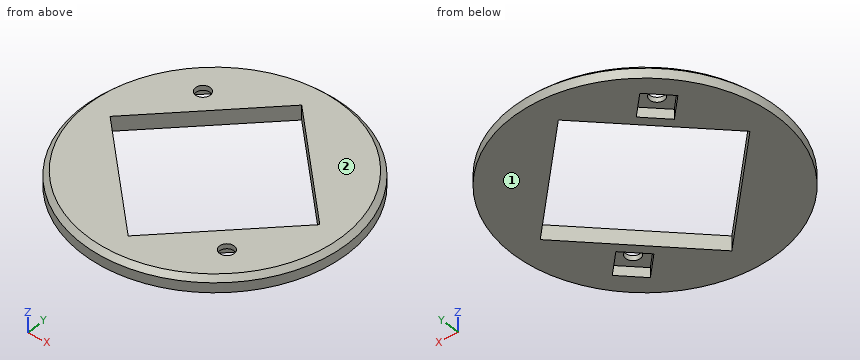
from build123d import *

# Parameters (mm, degrees)
BOX318_W                    = 6
BOX318_H                    = 6
BOX318_DEPTH                = 20
BOX318_PLACEMENT_ANGLE      = 45
BOX319_W                    = 6
BOX319_H                    = 6
BOX319_DEPTH                = 20
BOX319_PLACEMENT_ANGLE      = 135
CYLINDER809_R               = 1.5
CYLINDER809_DEPTH           = 20
CYLINDER809_PLACEMENT_ANGLE = 135
CYLINDER808_R               = 1.5
CYLINDER808_DEPTH           = 20
CYLINDER808_PLACEMENT_ANGLE = 45
BOX315_W                    = 30.2
BOX315_H                    = 30.2
BOX315_DEPTH                = 100
BOX315_PLACEMENT_ANGLE      = 45
CYLINDER805_R               = 27
CYLINDER805_DEPTH           = 3
CHAMFER_SIZE                = 1


with BuildPart() as krychle318:
    # Box318 → Box318 (new body)
    with BuildSketch(Plane.XY):
        with Locations((3, 3)):
            Rectangle(BOX318_W, BOX318_H)
    extrude(amount=BOX318_DEPTH)


with BuildPart() as krychle318_1:
    # Box318 placement: moved
    add(krychle318.part.moved(Location((9.899495, -14.142136, -30))).rotate(Axis((9.899495, -14.142136, -30), (0, 0, -1)), BOX318_PLACEMENT_ANGLE))


with BuildPart() as compound722:
    # Box319 → Box319 (new body)
    with BuildSketch(Plane.XY):
        with Locations((3, 3)):
            Rectangle(BOX319_W, BOX319_H)
    extrude(amount=BOX319_DEPTH)


with BuildPart() as compound722_1:
    # Box319 placement: moved
    add(compound722.part.moved(Location((-9.899495, 14.142136, -30))).rotate(Axis((-9.899495, 14.142136, -30), (0, 0, 1)), BOX319_PLACEMENT_ANGLE))

    # Compound722: union Krychle318
    add(krychle318_1.part)


with BuildPart() as compound722_2:
    # Compound722 placement: moved
    add(compound722_1.part.moved(Location((0, 0, -13))))


with BuildPart() as obj1:
    # Cylinder809 → Cylinder809 (new body)
    with BuildSketch(Plane.XY):
        Circle(CYLINDER809_R)
    extrude(amount=CYLINDER809_DEPTH)


with BuildPart() as obj1_1:
    # Cylinder809 placement: moved
    add(obj1.part.moved(Location((-14.142136, 14.142136, -30))).rotate(Axis((-14.142136, 14.142136, -30), (0, 0, 1)), CYLINDER809_PLACEMENT_ANGLE))


with BuildPart() as compound:
    # Cylinder808 → Cylinder808 (new body)
    with BuildSketch(Plane.XY):
        Circle(CYLINDER808_R)
    extrude(amount=CYLINDER808_DEPTH)


with BuildPart() as compound_1:
    # Cylinder808 placement: moved
    add(compound.part.moved(Location((14.142136, -14.142136, -30))).rotate(Axis((14.142136, -14.142136, -30), (0, 0, -1)), CYLINDER808_PLACEMENT_ANGLE))

    # Compound: union obj1
    add(obj1_1.part)


with BuildPart() as krychle315:
    # Box315 → Box315 (new body)
    with BuildSketch(Plane.XY):
        with Locations((15.1, 15.1)):
            Rectangle(BOX315_W, BOX315_H)
    extrude(amount=BOX315_DEPTH)


with BuildPart() as krychle315_1:
    # Box315 placement: moved
    add(krychle315.part.moved(Location((0, -21.354625, -30))).rotate(Axis((0, -21.354625, -30), (0, 0, 1)), BOX315_PLACEMENT_ANGLE))


with BuildPart() as cut344:
    # Cylinder805 → Cylinder805 (new body)
    with BuildSketch(Plane.XY.offset(-25)):
        Circle(CYLINDER805_R)
    extrude(amount=CYLINDER805_DEPTH)

    # Chamfer
    chamfer_edges = [cut344.edges().sort_by_distance(p)[0] for p in [
        (-27, 0, -22),
    ]]
    chamfer(chamfer_edges, length=CHAMFER_SIZE)

    # Cut340: cut Krychle315
    add(krychle315_1.part, mode=Mode.SUBTRACT)

    # Cut342: cut Compound
    add(compound_1.part, mode=Mode.SUBTRACT)

    # Cut344: cut Compound722
    add(compound722_2.part, mode=Mode.SUBTRACT)


solid = cut344.part
Geometry: final body of the model. Coordinates: model frame, mm. Face numbers are marked on the shaded views. Coordinates: 2 decimals unless noted, no trailing zeros. Order: outer loops, then holes, each group sorted by start corner. A loop starts at its lowest first (then second) coordinate and runs counter-clockwise, first axis right, second up. Notation, with made-up numbers: (-18.5, 27.25) - (29.5, 27.25) arc R16 cw to (29.5, 48.25) - close; hole circle Ø9 at (74, 86.5). An arc over 180 degrees is marked (long way). Use one line per item in the form item = value.
1) Ray query, L1, parallel to X at y = 13, z = -22.55; L2, parallel to X at y = 14, z = -24; L3, parallel to Y at x = 13, z = -23.6. Return the intervals inside material, ascending.
Solutions:
L1 = -23.15 to -15.11, -13.17 to -8.35, 8.35 to 23.15
L2 = -23.09 to -18.24, -10.04 to -7.35, 7.35 to 23.09
L3 = -23.66 to -17.24, -11.04 to -8.35, 8.35 to 23.66
2) Section A-A (z = -23.6). Return loops of the section in (x, y), then the cut area to 3 significant figures.
Solutions:
outline = circle Ø54 at (0, 0); hole (-21.35, 0) - (0, -21.35) - (21.35, 0) - (0, 21.35) - close; hole (-18.38, 14.14) - (-14.14, 9.9) - (-9.9, 14.14) - (-14.14, 18.38) - close; hole (9.9, -14.14) - (14.14, -18.38) - (18.38, -14.14) - (14.14, -9.9) - close
area = 1,310 mm^2
3) Mould query, pull axis Z, two halves, no side actions, for the marked faces 1 and 2. Classes: +Z half, -Z half, draft (parallel to the pull), parting line (faces both ways), or undercut.
Solutions:
face_1 = -Z half
face_2 = +Z half
